Verification items for the finished model (mm, model axes). Face numbers are marked on the shaded views. Round coordinates to 2 decimals unless told otherwise and drop trailing zeros. Order: outer loops, then holes, each group sorted by start corner. A loop starts at its lowest first (then second) coordinate and runs counter-clockwise, first axis right, second up. Notation, with made-up numbers: (14, 88.25) -> (22, 88.25) arc R23 ccw to (22, 105.25) -> close; hole circle Ø1 at (3, 14.25). An arc over 180 degrees is marked (long way). Put each result on its own line as item: value.
```python
from build123d import *

# Parameters (mm, degrees)
SKETCH1_W           = 16
SKETCH1_H           = 3.5
BOSS_EXTRUDE1_START = -7
SKETCH3_R           = 1.375
BOSS_EXTRUDE1_DEPTH = 2.5
SKETCH4_R           = 2
BOSS_EXTRUDE2_DEPTH = 16


with BuildPart() as part:
    # Sketch1 → Revolve1 (revolve)
    with BuildSketch(Plane(origin=(0, 0, 0), x_dir=(1, 0, 0), z_dir=(0, 1, 0)), mode=Mode.PRIVATE) as revolve1_sk:
        with Locations((8, 17.75)):
            Rectangle(SKETCH1_W, SKETCH1_H)
    revolve(revolve1_sk.sketch.rotate(Axis((0, 0, 0), (1, 0, 0)), 180), axis=Axis((0, 0, 0), (1, 0, 0)))

    # Sketch2 → Cut-Revolve1 (revolve, cut)
    with BuildSketch(Plane(origin=(0, 0, 0), x_dir=(1, 0, 0), z_dir=(0, 1, 0)), mode=Mode.PRIVATE) as cut_revolve1_sk:
        Polygon((16, 17.5), (13.5, 17.5), (11, 16), (16, 16), align=None)
    revolve(cut_revolve1_sk.sketch.rotate(Axis((0, 0, 0), (1, 0, 0)), 180), axis=Axis((0, 0, 0), (1, 0, 0)), mode=Mode.SUBTRACT)

    # Sketch3 → Boss-Extrude1 (add)
    with BuildSketch(Plane.ZY.offset(BOSS_EXTRUDE1_START)):
        with Locations((0, 16)):
            Circle(SKETCH3_R)
        with Locations((16, 0)):
            Circle(SKETCH3_R)
        with Locations((0, -16)):
            Circle(SKETCH3_R)
        with Locations((-16, 0)):
            Circle(SKETCH3_R)
    extrude(amount=-BOSS_EXTRUDE1_DEPTH)

    # Sketch4 → Boss-Extrude2 (add)
    with BuildSketch(Plane.ZY):
        with Locations((0, 19.5)):
            Circle(SKETCH4_R)
        with Locations((19.5, 0)):
            Circle(SKETCH4_R)
        with Locations((0, -19.5)):
            Circle(SKETCH4_R)
        with Locations((-19.5, 0)):
            Circle(SKETCH4_R)
    extrude(amount=-BOSS_EXTRUDE2_DEPTH)


solid = part.part
```
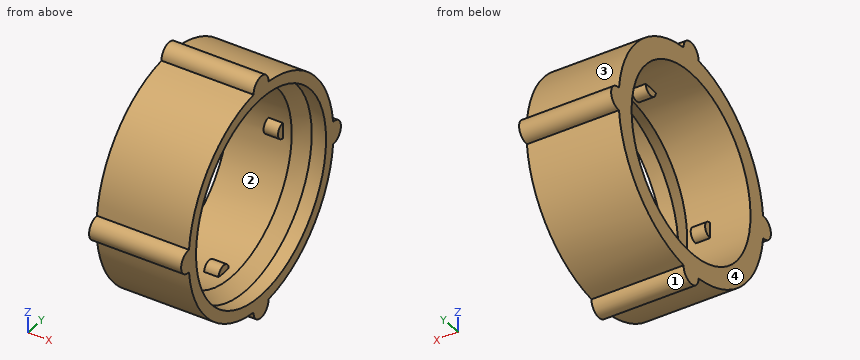
Item 1: Depth check by flat-ended pin: pin 1 Ø3 at (x, z) = (12, -4.5) entering from +Y; pin 2 Ø1 at (x, y) = (4.5, 14.5) entering from -Z; pin 3 Ø5 at (x, y) = (11.5, -16) entering from +Z. Enter the tip coordinate at first touch or a pass-through.
Geometry check:
pin 1: y = 19.27
pin 2: z = -13.57
pin 3: z = 14.07
Item 2: Sectioned sample at B-B, the plane x = 6. Record the boundary of the cut face in (y, z).
Geometry check:
outline: (-19.4, -2) arc R19.5 ccw to (-2, -19.4) arc R2 ccw (long way) to (2, -19.4) arc R19.5 ccw to (19.4, -2) arc R2 ccw (long way) to (19.4, 2) arc R19.5 ccw to (2, 19.4) arc R2 ccw (long way) to (-2, 19.4) arc R19.5 ccw to (-19.4, 2) arc R2 ccw (long way) to start; hole circle Ø32 at (0, 0)
Item 3: Release check for a two-part mould opening along Y. For the marked faces 1, 2, 3 and 4 record: pulls with the +Y half, pulls with the -Y half, needs draft (parallel to the pull), parting line crosses it, or undercut.
Geometry check:
face 1: parting line crosses it
face 2: undercut
face 3: pulls with the +Y half
face 4: needs draft
Item 4: Sectioned sample at A-A, the plane x = 14.75. Record the boundary of the cut face in (y, z).
Geometry check:
outline: (-19.4, -2) arc R19.5 ccw to (-2, -19.4) arc R2 ccw (long way) to (2, -19.4) arc R19.5 ccw to (19.4, -2) arc R2 ccw (long way) to (19.4, 2) arc R19.5 ccw to (2, 19.4) arc R2 ccw (long way) to (-2, 19.4) arc R19.5 ccw to (-19.4, 2) arc R2 ccw (long way) to start; hole circle Ø35 at (0, 0)
Item 5: Material ranges on line 1 along Y through (x, z) = (3.5, 0); line 2 along Y through (x, z) = (15, 0); line 3 along Z through (x, y) = (12, -3), recorded low to high.
Geometry check:
line 1: -21.5 to -16, 16 to 21.5
line 2: -21.5 to -17.5, 17.5 to 21.5
line 3: -19.27 to -16.33, 16.33 to 19.27
